```python
from build123d import *

# Parameters (mm, degrees)
SKETCH1_R               = 24.53
BOSS_EXTRUDE1_DEPTH     = 22.008152455
CUT_EXTRUDE3_DEPTH      = 23.008152455
CUT_EXTRUDE3_DEPTH_BACK = 1


with BuildPart() as part:
    # Sketch1 → Boss-Extrude1 (new body)
    with BuildSketch(Plane.XY):
        Circle(SKETCH1_R)
    extrude(amount=BOSS_EXTRUDE1_DEPTH)

    # Sketch2 → Cut-Extrude3 (cut, two sides)
    with BuildSketch(Plane.XY) as cut_extrude3_sk:
        with BuildLine():
            Line((20.955145444, 0), (19.5125, 0))
            ThreePointArc((19.5125, 0), (19.473005706, -1.240848518), (19.354682699, -2.476673954))
            Line((19.354682699, -2.476673954), (20.785660011, -2.659785415))
            add(Edge.make_bspline(
                [(20.785660011, -2.659785415), (20.800985299, -2.662076983), (20.843806968, -2.669507053), (20.924073429, -2.687499122), (21.05378572, -2.72241867), (21.216979197, -2.774995556), (21.425137234, -2.852162258), (21.666388368, -2.954705307), (21.926945547, -3.07951949), (22.20493909, -3.228005325), (22.477187641, -3.387439173), (22.743526717, -3.556434161), (23.004180465, -3.734229594), (23.313555372, -3.959446459), (23.619528341, -4.200366277), (23.856411219, -4.400665356), (24.029365424, -4.554471972), (24.092590531, -4.611722182)],
                knots=[0, 0, 0, 0, 0, 0.005376748, 0.015083688, 0.02853182, 0.046610139, 0.064854849, 0.092110525, 0.119476175, 0.146842495, 0.174208853, 0.201574955, 0.228941013, 0.256307345, 0.307035032, 0.336633369, 0.336633369, 0.336633369, 0.336633369, 0.336633369], degree=4))
            ThreePointArc((24.092590531, -4.611722182), (24.420402799, -2.316209648), (24.53, 0))
            ThreePointArc((24.53, 0), (24.518268205, 0.75856723), (24.483084041, 1.51640887))
            add(Edge.make_bspline(
                [(20.955145444, 0), (20.970637643, 0.000327832), (21.014056051, 0.002262558), (21.095957005, 0.009921081), (21.229052435, 0.028094135), (21.397599457, 0.059532029), (21.613868491, 0.109653615), (21.866183922, 0.180745878), (22.140476071, 0.271478677), (22.435068144, 0.383478516), (22.725351294, 0.507067017), (23.010986338, 0.640889404), (23.292099055, 0.784162682), (23.627557961, 0.96828979), (23.961635582, 1.168424644), (24.222026021, 1.337036737), (24.413103669, 1.467646709), (24.483084041, 1.51640887)],
                knots=[0, 0, 0, 0, 0, 0.005376748, 0.015083688, 0.02853182, 0.046610139, 0.064854849, 0.092110525, 0.119476175, 0.146842495, 0.174208853, 0.201574955, 0.228941013, 0.256307345, 0.307035032, 0.336633369, 0.336633369, 0.336633369, 0.336633369, 0.336633369], degree=4))
        make_face()
    extrude(amount=CUT_EXTRUDE3_DEPTH, mode=Mode.SUBTRACT)
    extrude(cut_extrude3_sk.sketch, amount=-CUT_EXTRUDE3_DEPTH_BACK, mode=Mode.SUBTRACT)


solid = part.part
```
Read the model definition and answer for the solid it produces. Units are mm, in the model's axes. A direction names the side the tool comes from. Give positions to 0.01 mm unless a question says otherwise; leave off trailing zeros. Write each loop counter-clockwise with the first axis right and the second up, starting at its lowest first coordinate (ties: lowest second). Pieces come first, ordered by that corner, then holes. Notation, with made-up numbers: (-13, -26.75) -> (10, -26.75) arc R18 ccw to (10, 8.25) -> close; hole circle Ø9 at (-28, 40.5). An arc over 180 degrees is marked (long way). Answer in a Markdown table with one row per item.
1) Straight lines are drawn through the part: line 1 (Y direction, x = 21, z = 6); line 2 (Y direction, x = 22.5, z = 7.5); line 3 (X direction, y = -6.5, z = 9.75). For each, find the intervals that lie inside material, in ascending order. Write a range as [from, to].
Results list:
| item | result |
|---|---|
| line 1 | [-12.68, -2.71], [0, 12.68] |
| line 2 | [-9.77, -3.4], [0.41, 9.77] |
| line 3 | [-23.65, 23.65] |
2) Section A-A on y = -17.5 is taken. Give the vertices of the cut face in (x, z).
Results list:
| item | result |
|---|---|
| outline | (-17.19, 0) -> (17.19, 0) -> (17.19, 22.01) -> (-17.19, 22.01) -> close |
3) Section B-B on x = -5.5 is taken. Give the vertices of the cut face in (y, z), plus the area to 3 significant figures.
Results list:
| item | result |
|---|---|
| outline | (-23.91, 0) -> (23.91, 0) -> (23.91, 22.01) -> (-23.91, 22.01) -> close |
| area | 1,050 mm^2 |
4) Determine the mould class of faces 1 (the cylindrical face through (19.474, -1.223, 10.85)), 2 (the flat face through (20.06, -2.567, 10.85)), 3 (the flat face through (0, 0, 22.008)), 4 (the cylindrical face through (-24.393, 2.592, 10.85)) for opening direction Y: released by +Y, released by -Y, zero draft, split by the parting line, or undercut.
Results list:
| item | result |
|---|---|
| face 1 | undercut |
| face 2 | undercut |
| face 3 | zero draft |
| face 4 | split by the parting line |
5) A tool of negligible diameter and unlimited length cuts with its end or side. For faces 5 (the flat face through (0, 0, 0)), 6 (the flat face through (20, 0, 11)), from which of +Z, -Z, +X, -X, +Y, -Y can it reach the whole face along a straight path? Write none if from no direction.
Results list:
| item | result |
|---|---|
| face 5 | -Z, +X, -X, +Y, -Y |
| face 6 | +Z, -Z, +X |
6) Each of these flat-tipped pins is pushed along its axis until it touches: pin 1 Ø0.7 at (x, z) = (20.5, 15) entering from -Y; pin 2 Ø5 at (y, z) = (15.5, 6.5) entering from -X; pin 3 Ø10 at (x, z) = (-13, 11) entering from -Y. Where does it stop, or does it pass through?
Results list:
| item | result |
|---|---|
| pin 1 | y = -13.99 |
| pin 2 | x = -20.8 |
| pin 3 | y = -23.19 |
